Work out the finished part from the listing and answer in its coordinate system (mm). A direction names the side the tool comes from. Round coordinates to 2 decimals unless told otherwise and drop trailing zeros. Write each loop counter-clockwise with the first axis right and the second up, starting at its lowest first coordinate (ties: lowest second). Pieces come first, ordered by that corner, then holes. Notation, with made-up numbers: (73, -27) -> (129, -27) arc R17 cw to (129, -17) -> close; hole circle Ø10 at (47.5, -1.75). An arc over 180 degrees is marked (long way). One line per item, written item: value.
```python
from build123d import *

# Parameters (mm, degrees)
F0_W      = 54
F0_H      = 39
F1_DEPTH  = 13
F2_W      = 50.5
F2_H      = 35.5
F3_DEPTH  = 8
F4_W      = 24
F4_H      = 24
F5_DEPTH  = 3
F6_W      = 21
F6_H      = 21
F7_DEPTH  = 2
F8_R      = 5
F9_R      = 7
F10_W     = 4.5
F10_H     = 1.5
F11_DEPTH = 1.75


with BuildPart() as f1:
    # F0 (on Top) → F1 (new body)
    with BuildSketch(Plane.XY):
        Rectangle(F0_W, F0_H)
    extrude(amount=F1_DEPTH)

    # F2 (on face) → F3 (cut)
    with BuildSketch(Plane.XY.offset(13)):
        Rectangle(F2_W, F2_H)
    extrude(amount=-F3_DEPTH, mode=Mode.SUBTRACT)

    # F4 (on face) → F5 (cut)
    with BuildSketch(Plane(origin=(0, 0, 0), x_dir=(1, 0, 0), z_dir=(0, 0, -1))):
        with Locations((-9.3, 0)):
            Rectangle(F4_W, F4_H)
    extrude(amount=-F5_DEPTH, mode=Mode.SUBTRACT)

    # F6 (on face) → F7 (cut)
    with BuildSketch(Plane(origin=(0, 0, 3), x_dir=(1, 0, 0), z_dir=(0, 0, -1))):
        with Locations((-9.329, -0.501032)):
            Rectangle(F6_W, F6_H)
    extrude(amount=-F7_DEPTH, mode=Mode.SUBTRACT)

    # F8
    f8_edges = [f1.edges().sort_by_distance(p)[0] for p in [
        (-25.25, 17.75, 9),
        (25.25, 17.75, 9),
        (-25.25, -17.75, 9),
        (25.25, -17.75, 9),
    ]]
    fillet(f8_edges, radius=F8_R)

    # F9
    f9_edges = [f1.edges().sort_by_distance(p)[0] for p in [
        (-27, 19.5, 6.5),
        (-27, -19.5, 6.5),
        (27, 19.5, 6.5),
        (27, -19.5, 6.5),
    ]]
    fillet(f9_edges, radius=F9_R)

    # F10 (on face) → F11 (cut)
    with BuildSketch(Plane.YZ.offset(27)):
        with Locations((0, 5.75)):
            Rectangle(F10_W, F10_H)
    extrude(amount=-F11_DEPTH, mode=Mode.SUBTRACT)


solid = f1.part
```
(1) Find section A-A on x = -17. Give the vertices of the cut face in (y, z).
Reported:
outline: (-19.5, 0) -> (-12, 0) -> (-12, 3) -> (-10, 3) -> (-10, 5) -> (-17.75, 5) -> (-17.75, 13) -> (-19.5, 13) -> close; (11, 3) -> (12, 3) -> (12, 0) -> (19.5, 0) -> (19.5, 13) -> (17.75, 13) -> (17.75, 5) -> (11, 5) -> close
(2) Consider probe 1 along X at (y, z) = (3, 1.75); probe 2 along X at (y, z) = (5, 6); probe 3 along Y at (x, z) = (-11, 11). Determine where each line is inside the solid, lowest interval first.
Reported:
probe 1: x = -27 to -21.3, 2.7 to 27
probe 2: x = -27 to -25.25, 25.25 to 27
probe 3: y = -19.5 to -17.75, 17.75 to 19.5
(3) For a pull along X with two mould halves and no side action, classify faces 4 (the face through (27, 0, 8)), 5 (the face through (26, 2.25, 6)), 6 (the face through (-25.25, 0, 9)) as pulls with the +X half, pulls with the -X half, needs draft (parallel to the pull), parting line crosses it, or undercut.
Reported:
face 4: pulls with the +X half
face 5: needs draft
face 6: undercut
(4) Find section C-C on z = 7.5. Give the vertices of the cut face in (x, y), plus the area to 3 significant figures.
Reported:
outline: (-27, -12.5) arc R7 ccw to (-20, -19.5) -> (20, -19.5) arc R7 ccw to (27, -12.5) -> (27, 12.5) arc R7 ccw to (20, 19.5) -> (-20, 19.5) arc R7 ccw to (-27, 12.5) -> close; hole (-25.25, -12.75) arc R5 ccw to (-20.25, -17.75) -> (20.25, -17.75) arc R5 ccw to (25.25, -12.75) -> (25.25, 12.75) arc R5 ccw to (20.25, 17.75) -> (-20.25, 17.75) arc R5 ccw to (-25.25, 12.75) -> close
area: 293 mm2
(5) Find section B-B on y = -3. Give the vertices of the cut face in (x, z).
Reported:
outline: (-27, 0) -> (-21.3, 0) -> (-21.3, 3) -> (-19.83, 3) -> (-19.83, 5) -> (-25.25, 5) -> (-25.25, 13) -> (-27, 13) -> close; (1.17, 3) -> (2.7, 3) -> (2.7, 0) -> (27, 0) -> (27, 13) -> (25.25, 13) -> (25.25, 5) -> (1.17, 5) -> close
(6) A tool of negligible diameter and unlimited length cuts with its end or side. For faces 1 (the face through (-21.3, 0, 1)), 2 (the face through (23.82, 16.25, 8.94)), 3 (the face through (26, 0, 6.5)), from which of +Z, -Z, +X, -X, +Y, -Y can it reach the whole face along a straight path? Write none if from no direction.
Reported:
face 1: -Z
face 2: +Z
face 3: +X
(7) Flat-ended cylindrical pins translate along their axes: pin 1 Ø4 at (x, y) = (-6.5, -15.5) entering from +Z; pin 2 Ø0.8 at (x, z) = (26, 5.5) entering from +Y; pin 3 Ø1.2 at (x, z) = (26, 6) entering from -Y; pin 4 Ø3 at (x, y) = (-5.5, -13.5) entering from -Z. Find the tip coordinate at first contact, or state that the pin passes through.
Reported:
pin 1: stops at z = 5
pin 2: stops at y = 16.7
pin 3: stops at y = -16.95
pin 4: stops at z = 0
(8) Find section D-D on y = 1.5. Give the vertices of the cut face in (x, z), plus the area to 3 significant figures.
Reported:
outline: (-27, 0) -> (-21.3, 0) -> (-21.3, 3) -> (-19.83, 3) -> (-19.83, 5) -> (-25.25, 5) -> (-25.25, 13) -> (-27, 13) -> close; (1.17, 3) -> (2.7, 3) -> (2.7, 0) -> (27, 0) -> (27, 5) -> (1.17, 5) -> close; (25.25, 6.5) -> (27, 6.5) -> (27, 13) -> (25.25, 13) -> close
area: 181 mm2
